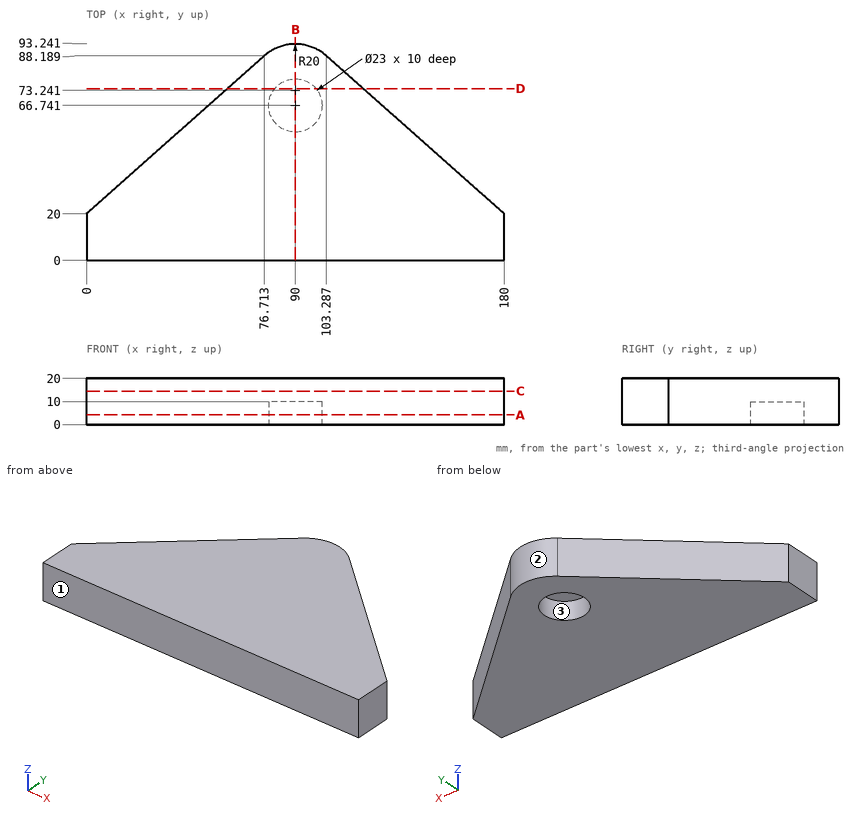
Check sheet for the drawn part. Datum: minimum x, y, z corner. Units: mm. Round coordinates to 2 decimals unless told otherwise and drop trailing zeros. Write each loop counter-clockwise with the first axis right and the second up, starting at its lowest first coordinate (ties: lowest second). Pieces come first, ordered by that corner, then holes. Notation, with made-up numbers: (-18, 20) -> (17, 20) arc R22 cw to (17, 56) -> close; hole circle Ø4 at (32, 9.5). An arc over 180 degrees is marked (long way). Write each question's results on one line, items separated by ' | '. Start each with the question number.
1. Cross-section at B-B (x = 90). Enter the section's corners in (y, z), then the cut area to 3 significant figures.
2. Cross-section at D-D (y = 74). Enter the section's corners in (x, z), then the cut area to 3 significant figures.
3. Draft check along Y on the marked faces 1, 2 and 3. Enter one of: +Y half, -Y half, draft (parallel to the pull), parting line (faces both ways), or undercut.
4. Cross-section at A-A (z = 4.25). Enter the section's corners in (x, y).
5. Material ranges on probe 1 along Y at (x, z) = (90, 2.75); probe 2 along X at (y, z) = (76.5, 7.25) (1 decimal); probe 3 along X at (y, z) = (77, 7.5) (1 decimal), recorded low to high. Write a range as from..to.
6. Depth check by flat-ended pin: P1, Ø4, axis at x = 29, z = 5, coming from the +Y side (1 decimal); P2, Ø5, axis at y = 23.5, z = 12.5, coming from the -X side (1 decimal); P3, Ø11.5, axis at x = 85.5, y = 69.5, coming from the -Z side. Enter the tip coordinate at first touch or a pass-through.
7. Cross-section at C-C (z = 14.5). Enter the section's corners in (x, y), then the cut area to 3 significant figures.
Solutions:
1) outline: (0, 0) -> (55.24, 0) -> (55.24, 10) -> (78.24, 10) -> (78.24, 0) -> (93.24, 0) -> (93.24, 20) -> (0, 20) -> close | area: 1,630 mm2
2) outline: (60.75, 0) -> (81.08, 0) -> (81.08, 10) -> (98.92, 10) -> (98.92, 0) -> (119.25, 0) -> (119.25, 20) -> (60.75, 20) -> close | area: 992 mm2
3) face 1: -Y half | face 2: +Y half | face 3: undercut
4) outline: (0, 0) -> (180, 0) -> (180, 20) -> (103.29, 88.19) arc R20 ccw to (76.71, 88.19) -> (0, 20) -> close; hole circle Ø23 at (90, 66.74)
5) probe 1: y = 0..55.24, 78.24..93.24 | probe 2: x = 63.6..83.9, 96.1..116.4 | probe 3: x = 64.1..84.8, 95.2..115.9
6) P1: stops at y = 47.6 | P2: stops at x = 1.1 | P3: stops at z = 10
7) outline: (0, 0) -> (180, 0) -> (180, 20) -> (103.29, 88.19) arc R20 ccw to (76.71, 88.19) -> (0, 20) -> close | area: 10,700 mm2
